For this review, use the dimensioned drawing (mm, ordinates from the lowest corner) and the shaded views. Give positions to 0.01 mm unless a question says otherwise; leave off trailing zeros. Order: outer loops, then holes, each group sorted by start corner. A loop starts at its lowest first (then second) coordinate and runs counter-clockwise, first axis right, second up. Notation, with made-up numbers: M 46.25,-10 L 58.25,-10 A17 ccw 58.25,-1 Z; hole C 46,77 d6. An arc over 180 degrees is marked long. Answer as CSV lines item,"result". Start each with the question number.
1. We need section C-C, the plane y = 3.25. Give the boundary of the cut face in (x, z).
2. For line 1 along Y through (x, z) = (39, 8); line 2 along Z through (x, y) = (19.5, 2.9); line 3 along X through (y, z) = (2.25, 22), list the stretches that pass through material, from the lowest coordinate up.
3. We need section D-D, the plane z = 9.75. Give the boundary of the cut face in (x, y), and give its area (3 significant figures).
4. We need section B-B, the plane x = 32.5. Give the boundary of the cut face in (y, z).
5. Clearance check with flat-ended pins moving along their axes: P1, Ø3, axis at x = 27.5, y = 4, coming from the +Z side; P2, Ø0.8, axis at x = 25, y = 3.5, coming from the -Z side; P3, Ø0.8, axis at y = 4, z = 12, coming from the -X side. State where each tip first meets the part, or that it passes through.
6. We need section A-A, the plane z = 12.25. Give the boundary of the cut face in (x, y), and give its area (3 significant figures).
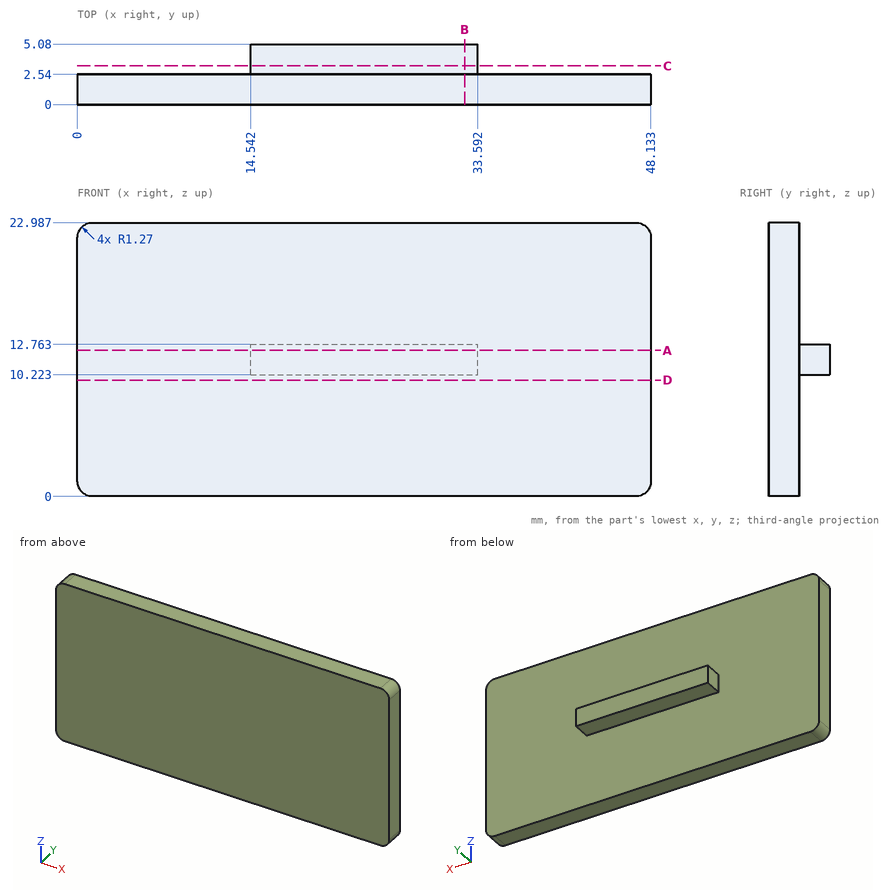
Result set:
1,outline,"M 14.54,10.22 L 33.59,10.22 L 33.59,12.76 L 14.54,12.76 Z"
2,line 1,"0 to 2.54"
2,line 2,"10.22 to 12.76"
2,line 3,"0.03 to 48.1"
3,outline,"M 0,0 L 48.13,0 L 48.13,2.54 L 0,2.54 Z"
3,area,"122 mm2"
4,outline,"M 0,0 L 2.54,0 L 2.54,10.22 L 5.08,10.22 L 5.08,12.76 L 2.54,12.76 L 2.54,22.99 L 0,22.99 Z"
5,P1,"z = 22.99"
5,P2,"z = 10.22"
5,P3,"x = 14.54"
6,outline,"M 0,0 L 48.13,0 L 48.13,2.54 L 33.59,2.54 L 33.59,5.08 L 14.54,5.08 L 14.54,2.54 L 0,2.54 Z"
6,area,"171 mm2"
